Can you work these out from the model? Positions are in its coordinate system, mm. A direction names the side the tool comes from. Round coordinates to 2 decimals unless told otherwise and drop trailing zeros. Answer as CSV lines item,"result". Start each with the question number.
from build123d import *

# Parameters (mm, degrees)
SKETCH2_R           = 5
SKETCH2_R_2         = 1.75
BOSS_EXTRUDE1_DEPTH = 8.5
BOSS_EXTRUDE2_START = -8.5
BOSS_EXTRUDE2_DEPTH = 8.5


with BuildPart() as part:
    # Sketch2 → Boss-Extrude1 (new body)
    # profile 1 of 3: a face of its own
    with BuildSketch(Plane(origin=(0, 0, 0), x_dir=(1, 0, 0), z_dir=(0, 1, 0))):
        Circle(SKETCH2_R)
        with Locations(Location((0, 0, 0), (0, 0, 270))):
            Circle(SKETCH2_R_2, mode=Mode.SUBTRACT)
    # profile 2 of 3: a face of its own
    with BuildSketch(Plane(origin=(0, 0, 0), x_dir=(1, 0, 0), z_dir=(0, 1, 0))):
        with BuildLine():
            Line((22, 5), (0, 5))
            ThreePointArc((0, 5), (3.535533906, 3.535533906), (5, 0))
            ThreePointArc((5, 0), (3.535533906, -3.535533906), (0, -5))
            Line((0, -5), (22, -5))
            ThreePointArc((22, -5), (17, 0), (22, 5))
        make_face()
    # profile 3 of 3: a face of its own
    with BuildSketch(Plane(origin=(0, 0, 0), x_dir=(1, 0, 0), z_dir=(0, 1, 0))):
        with Locations((22, 0)):
            Circle(SKETCH2_R)
        with Locations(Location((22, 0, 0), (0, 0, 270))):
            Circle(SKETCH2_R_2, mode=Mode.SUBTRACT)
    extrude(amount=BOSS_EXTRUDE1_DEPTH)

    # Sketch3 → Boss-Extrude2 (add)
    with BuildSketch(Plane(origin=(0, 8.5, 0), x_dir=(1, 0, 0), z_dir=(0, 1, 0)).offset(BOSS_EXTRUDE2_START)):
        with BuildLine():
            ThreePointArc((22, 5), (27, 0), (22, -5))
            Line((22, -5), (24.765014751, -5))
            Line((24.765014751, -5), (31.381419164, -1.772963949))
            add(Edge.make_bspline(
                [(31.381419164, -1.772963949), (41.129259451, 6.582699459), (53.966862985, 6)],
                knots=[0, 0, 0, 1, 1, 1], degree=2))
            Line((53.966862985, 6), (61.095847858, 9.630092929))
            Line((61.095847858, 9.630092929), (58.75, 12.87))
            add(Edge.make_bspline(
                [(12.956629398, 5), (32.247892428, 5.420652932), (42.340471259, 18.148408487), (58.75, 12.87)],
                knots=[0.03219955, 0.03219955, 0.03219955, 0.03219955, 1, 1, 1, 1], degree=3))
            Line((12.956629398, 5), (22, 5))
        make_face()
    extrude(amount=BOSS_EXTRUDE2_DEPTH)


solid = part.part
(1) I'm going to push flat-ended pins straight in: P1, Ø3, axis at y = 4.5, z = -2, coming from the -X side; P2, Ø1, axis at y = 2.5, z = -4.5, coming from the -X side. Where does each tip first touch, or does it pass through?
(2) For faces 4 (the flat face through (59.939, 4.19, -11.227)), 5 (the flat face through (7, 4, -5)), which set-ups out of +Z, -Z, +X, -X, +Y, -Y let a thin tool reach every point of the face, with its end or its side?
(3) If I drill on line 1 along X through (y, z) = (2, 0); line 2 along Z through (x, y) = (23, 3); line 3 along Z through (x, y) = (3.5, 8.25), over which ranges is the centre line in solid material (lowest first)?
(4) I want a section at A-A on y = 3.25. Count the separate pieces of the cut face and the enclosed holes in it, and give its area (3 significant figures).
(5) If we mould it in two halves opening along Z, with no side actions, what happens to faces 1 (the flat face through (28.027, 4.19, 3.409)), 2 (the cylindrical face through (23.735, 4.19, -0.228)), 3 (the flat face through (28, 0, -4))? For each: +Z half, -Z half, draft (parallel to the pull), parting line (faces both ways), or undercut.
From the geometry:
1,P1,"x = -4.97"
1,P2,"x = -3"
2,face 4,"-Z, +X, +Y, -Y"
2,face 5,"-Z, -X, +Y, -Y"
3,line 1,"-5 to -1.75, 1.75 to 20.25, 23.75 to 33.62"
3,line 2,"-6.35 to -1.44, 1.44 to 5"
3,line 3,"-5 to 5"
4,separate pieces,"1"
4,enclosed holes,"2"
4,area,"581 mm²"
5,face 1,"+Z half"
5,face 2,"undercut"
5,face 3,"draft"
